from build123d import *

# Parameters (mm, degrees)
SKETCH_1_R    = 2.6
SKETCH_1_R_2  = 1.3
M5_M2P5_DEPTH = 3


with BuildPart() as part:
    # 草图1 → M5转接毂_双M2p5折叠轴孔 (new body)
    with BuildSketch(Plane.XY):
        Polygon((-9, -6), (9, -6), (13, -2), (13, 2), (9, 6), (-9, 6), (-13, 2), (-13, -2), align=None)
        Circle(SKETCH_1_R, mode=Mode.SUBTRACT)
        with Locations((-8, 0)):
            Circle(SKETCH_1_R_2, mode=Mode.SUBTRACT)
        with Locations((8, 0)):
            Circle(SKETCH_1_R_2, mode=Mode.SUBTRACT)
    extrude(amount=M5_M2P5_DEPTH)


solid = part.part
The model under review builds one solid part; all positions refer to its coordinate system, in mm. Coordinates: 2 decimals unless noted, no trailing zeros. Write each loop counter-clockwise with the first axis right and the second up, starting at its lowest first coordinate (ties: lowest second). Pieces come first, ordered by that corner, then holes. Notation, with made-up numbers: (48, 30) -> (101, 30) arc R24 ccw to (101, 66) -> close; hole circle Ø7 at (40, -14.75). An arc over 180 degrees is marked (long way). Answer in a Markdown table with one row per item.
1. Draft analysis for pull direction X (two halves, no side actions). For faces 1 (the cylindrical face through (-0.338, 2.578, 1.479)), 2 (the flat face through (-11, 4, 1)), 3 (the flat face through (11, -4, 1)), 4 (the flat face through (0, 3, 3)), state which applies: +X half, -X half, draft (parallel to the pull), parting line (faces both ways), or undercut.
Answers below:
| item | result |
|---|---|
| face 1 | undercut |
| face 2 | -X half |
| face 3 | +X half |
| face 4 | draft |
2. We need section C-C, the plane z = 2.3. State the section outline as (x, y) points.
Answers below:
| item | result |
|---|---|
| outline | (-13, -2) -> (-9, -6) -> (9, -6) -> (13, -2) -> (13, 2) -> (9, 6) -> (-9, 6) -> (-13, 2) -> close; hole circle Ø2.6 at (-8, 0); hole circle Ø5.2 at (0, 0); hole circle Ø2.6 at (8, 0) |
3. Clearance check with a flat-ended pin moving along its axis: pin 1 Ø1.5 at (y, z) = (-3, 1.5) entering from +X. State where the tip first meets the part, or that it passes through.
Answers below:
| item | result |
|---|---|
| pin 1 | stops at x = 12.75 |
4. Wall thickness on probe 1 along Y at (x, z) = (8, 0.95); probe 2 along Y at (x, z) = (0, 1.35); probe 3 along X at (y, z) = (1, 1.7): over which ranges is each line inside the solid? List them lowest first. Write a range as [from, to].
Answers below:
| item | result |
|---|---|
| probe 1 | y = [-6, -1.3], [1.3, 6] |
| probe 2 | y = [-6, -2.6], [2.6, 6] |
| probe 3 | x = [-13, -8.83], [-7.17, -2.4], [2.4, 7.17], [8.83, 13] |
5. We need section A-A, the plane x = 8. State the section outline as (y, z) points, and give its area (3 significant figures).
Answers below:
| item | result |
|---|---|
| outline | (-6, 0) -> (-1.3, 0) -> (-1.3, 3) -> (-6, 3) -> close; (1.3, 0) -> (6, 0) -> (6, 3) -> (1.3, 3) -> close |
| area | 28.2 mm^2 |
6. We need section D-D, the plane x = 0. State the section outline as (y, z) points, and give its area (3 significant figures).
Answers below:
| item | result |
|---|---|
| outline | (-6, 0) -> (-2.6, 0) -> (-2.6, 3) -> (-6, 3) -> close; (2.6, 0) -> (6, 0) -> (6, 3) -> (2.6, 3) -> close |
| area | 20.4 mm^2 |
7. We need section B-B, the plane y = 0. State the section outline as (x, z) points, and give its area (3 significant figures).
Answers below:
| item | result |
|---|---|
| outline | (-13, 0) -> (-9.3, 0) -> (-9.3, 3) -> (-13, 3) -> close; (-6.7, 0) -> (-2.6, 0) -> (-2.6, 3) -> (-6.7, 3) -> close; (2.6, 0) -> (6.7, 0) -> (6.7, 3) -> (2.6, 3) -> close; (9.3, 0) -> (13, 0) -> (13, 3) -> (9.3, 3) -> close |
| area | 46.8 mm^2 |
